The listing builds one solid part. Answer for the finished solid, in the listing's coordinates (mm). A direction names the side the tool comes from. Round coordinates to 2 decimals unless told otherwise and drop trailing zeros. Order: outer loops, then holes, each group sorted by start corner. A loop starts at its lowest first (then second) coordinate and runs counter-clockwise, first axis right, second up. Notation, with made-up numbers: (-37, 54.25) -> (11, 54.25) arc R24 cw to (11, 70.25) -> close; hole circle Ø1 at (79, -30.5). An arc over 180 degrees is marked (long way). Answer in a Markdown table with one row per item. Add a question column.
```python
from build123d import *

# Parameters (mm, degrees)
BOSS_EXTRUDE1_DEPTH = 8
SKETCH2_R           = 1.5
SKETCH2_R_2         = 5
CUT_EXTRUDE1_DEPTH  = 25
FILLET1_R           = 5
CUT_EXTRUDE2_DEPTH  = 25
SKETCH5_R           = 1.5
CUT_EXTRUDE3_DEPTH  = 25


with BuildPart() as part:
    # Sketch1 → Boss-Extrude1 (new body)
    with BuildSketch(Plane(origin=(0, 0, 0), x_dir=(1, 0, 0), z_dir=(0, 1, 0))):
        with BuildLine():
            Line((0, 0), (150, 0))
            ThreePointArc((150, 0), (187.320508076, 10), (150, 20))
            Line((150, 20), (0, 20))
            Line((0, 20), (0, 0))
        make_face()
    extrude(amount=BOSS_EXTRUDE1_DEPTH)

    # Sketch2 → Cut-Extrude1 (cut)
    with BuildSketch(Plane(origin=(0, 8, 0), x_dir=(1, 0, 0), z_dir=(0, 1, 0))):
        with Locations((167.097723626, 0.502612618)):
            Circle(SKETCH2_R)
        with Locations((167.543292526, 19.497387382)):
            Circle(SKETCH2_R)
        with Locations((175.318307977, 9.812392042)):
            Circle(SKETCH2_R)
        with Locations((159.322708175, 10.187607958)):
            Circle(SKETCH2_R)
        with Locations((167.320508076, 10)):
            Circle(SKETCH2_R_2)
    extrude(amount=-CUT_EXTRUDE1_DEPTH, mode=Mode.SUBTRACT)

    # Fillet1
    fillet1_edges = [part.edges().sort_by_distance(p)[0] for p in [
        (0, 4, -20),
        (150, 4, -20),
        (150, 4, 0),
        (0, 4, 0),
    ]]
    fillet(fillet1_edges, radius=FILLET1_R)

    # Sketch4 → Cut-Extrude2 (cut)
    with BuildSketch(Plane(origin=(0, 8, 0), x_dir=(1, 0, 0), z_dir=(0, 1, 0))):
        Polygon((96, 3), (100.99769729, 17), (103.99769729, 17), (99, 3), align=None)
        Polygon((21.99769729, 17), (17, 3), (14, 3), (18.99769729, 17), align=None)
        Polygon((30.99769729, 17), (26, 3), (23, 3), (27.99769729, 17), align=None)
        Polygon((39.99769729, 17), (35, 3), (32, 3), (36.99769729, 17), align=None)
        Polygon((48.99769729, 17), (44, 3), (41, 3), (45.99769729, 17), align=None)
        Polygon((57.99769729, 17), (53, 3), (50, 3), (54.99769729, 17), align=None)
        Polygon((66.99769729, 17), (62, 3), (59, 3), (63.99769729, 17), align=None)
        Polygon((75.99769729, 17), (71, 3), (68, 3), (72.99769729, 17), align=None)
        Polygon((84.99769729, 17), (80, 3), (77, 3), (81.99769729, 17), align=None)
        Polygon((93.99769729, 17), (89, 3), (86, 3), (90.99769729, 17), align=None)
        Polygon((106, 3), (110.99769729, 17), (113.99769729, 17), (109, 3), align=None)
        Polygon((116, 3), (120.99769729, 17), (123.99769729, 17), (119, 3), align=None)
        Polygon((126, 3), (130.99769729, 17), (133.99769729, 17), (129, 3), align=None)
        Polygon((136, 3), (140.99769729, 17), (143.99769729, 17), (139, 3), align=None)
    extrude(amount=-CUT_EXTRUDE2_DEPTH, mode=Mode.SUBTRACT)

    # Sketch5 → Cut-Extrude3 (cut)
    with BuildSketch(Plane(origin=(0, 8, 0), x_dir=(1, 0, 0), z_dir=(0, 1, 0))):
        with Locations((6.810101414, 17.5)):
            Circle(SKETCH5_R)
        with Locations((6.810101414, 2.5)):
            Circle(SKETCH5_R)
    extrude(amount=-CUT_EXTRUDE3_DEPTH, mode=Mode.SUBTRACT)


solid = part.part
```
1. The part is cut by section C-C (x = 155). Give the vertices of the cut face in (y, z).
2. For faces 1 (the cylindrical face through (149.5, 4.1, 0.5)), 2 (the flat face through (101.534, 4.056, -10.098)), determine the directions among +Z, -Z, +X, -X, +Y, -Y from which every point of the face is accessible in a straight line to the end or side of a thin tool.
3. Straight lines are drawn through the part: line 1 along Z through (x, y) = (160, 3); line 2 along Z through (x, y) = (67.5, 1.25); line 3 along X through (y, z) = (4, -17.5). For each, find the intervals that lie inside material, in ascending order.
4. The part is cut by section A-A (y = 3.75). Give the number of separate pieces and of enclosed holes in the cut face, then the cut area to 3 significant figures.
5. The mould has two halves that part along Z. Classify faces 3 (the flat face through (92, 4, -17)), 4 (the cylindrical face through (149.586, 4.056, -20.542)), 5 (the flat face through (43, 4, -3)), 6 (the flat face through (92, 0, -10)): released by +Z, released by -Z, zero draft, split by the parting line, or undercut.
6. The part is cut by section B-B (z = -24.5). Give the vertices of the cut face in (x, y), then the cut area to 3 significant figures.
7. Each of these flat-tipped pins is pushed along its axis until it touches: pin 1 (0.9 mm diameter, centred on x = 117, y = 2, fed in from -Z); pin 2 (2.5 mm diameter, centred on x = 122.5, y = 4, fed in from +Z); pin 3 (1.5 mm diameter, centred on x = 156, z = -14.5, fed in from -Y); pin 4 (2 mm diameter, centred on y = 6.5, z = -6.5, fed in from +X). Where does it stop, or does it pass through?
Report:
| question | item | result |
|---|---|---|
| 1 | outline | (0, -25.75) -> (8, -25.75) -> (8, 5.75) -> (0, 5.75) -> close |
| 2 | face 1 | +Z, -X, +Y, -Y |
| 2 | face 2 | +Y, -Y |
| 3 | line 1 | z = -28.61 to -11.53, -8.85 to 8.61 |
| 3 | line 2 | z = -20 to 0 |
| 3 | line 3 | x = 0.67 to 5.31, 8.31 to 185.86 |
| 4 | separate pieces | 1 |
| 4 | enclosed holes | 21 |
| 4 | area | 3,500 mm^2 |
| 5 | face 3 | undercut |
| 5 | face 4 | released by -Z |
| 5 | face 5 | undercut |
| 5 | face 6 | zero draft |
| 6 | outline | (153.55, 0) -> (181.1, 0) -> (181.1, 8) -> (153.55, 8) -> close |
| 6 | area | 220 mm^2 |
| 7 | pin 1 | stops at z = -20 |
| 7 | pin 2 | stops at z = 0 |
| 7 | pin 3 | stops at y = 0 |
| 7 | pin 4 | stops at x = 187.16 |
